```python
from build123d import *

# Parameters (mm, degrees)
BOSS_EXTRUDE1_DEPTH = 80
BOSS_EXTRUDE2_DEPTH = 350
BOSS_EXTRUDE3_DEPTH = 350
SKETCH4_R           = 11
CUT_EXTRUDE1_DEPTH  = 350


with BuildPart() as part:
    # Sketch1 → Boss-Extrude1 (new, symmetric)
    with BuildSketch(Plane.XY):
        Polygon((15, 15), (-15, 15), (-15, 35), (-45, 35), (-45, 25), (-25, 25), (-25, -25), (-45, -25), (-45, -35), (-15, -35), (-15, -15), (15, -15), (15, -35), (45, -35), (45, -25), (25, -25), (25, 25), (45, 25), (45, 35), (15, 35), align=None)
    extrude(amount=BOSS_EXTRUDE1_DEPTH, both=True)

    # Sketch2 → Boss-Extrude2 (add)
    with BuildSketch(Plane.XY.offset(80)):
        Polygon((-45, -25), (-45, -35), (-15, -35), (-15, 35), (-45, 35), (-45, 25), (-25, 25), (-25, -25), align=None)
        Polygon((15, 35), (45, 35), (45, 25), (25, 25), (25, -25), (45, -25), (45, -35), (15, -35), align=None)
    extrude(amount=BOSS_EXTRUDE2_DEPTH)

    # Sketch3 → Boss-Extrude3 (add)
    with BuildSketch(Plane(origin=(0, 0, -80), x_dir=(-1, 0, 0), z_dir=(0, 0, -1))):
        Polygon((-45, -25), (-45, -35), (-15, -35), (-15, 35), (-45, 35), (-45, 25), (-25, 25), (-25, -25), align=None)
        Polygon((45, 35), (15, 35), (15, -35), (45, -35), (45, -25), (25, -25), (25, 25), (45, 25), align=None)
    extrude(amount=BOSS_EXTRUDE3_DEPTH)

    # Sketch4 → Cut-Extrude1 (cut)
    with BuildSketch(Plane.ZY.offset(25)):
        with Locations(Location((-415, 0, 0), (0, 0, 270))):
            Circle(SKETCH4_R)
        with Locations(Location((415, 0, 0), (0, 0, 270))):
            Circle(SKETCH4_R)
    extrude(amount=-CUT_EXTRUDE1_DEPTH, mode=Mode.SUBTRACT)


solid = part.part
```
Can you work these out from the model? Positions are in its coordinate system, mm. A direction names the side the tool comes from. Coordinates: 2 decimals unless noted, no trailing zeros. Loops run counter-clockwise (first coordinate to the right, second up) from the corner with the lowest first, then second, coordinate; pieces in that order, holes last. Notation, with made-up numbers: (33.5, 23.5) -> (54.5, 23.5) arc R31 cw to (54.5, 60.5) -> close; hole circle Ø9 at (-21.75, 45.25). An arc over 180 degrees is marked (long way). Answer as a JSON object with one key per item and string values.
1) Thinking about a two-plate mould opening in Z: for faces 5 (the face through (-24, 0, 430)), 6 (the face through (19.93, 2.38, 404.26)), 7 (the face through (-35, -25, 6)), which applies, pulls with the +Z half, pulls with the -Z half, needs draft (parallel to the pull), parting line crosses it, or undercut?
Results:
{"face 5": "pulls with the +Z half", "face 6": "undercut", "face 7": "needs draft"}
2) For P1, Ø17.5, axis at y = 0, z = -415, coming from the +X side; P2, Ø21, axis at y = -8, z = 117.5, coming from the +X side; P3, Ø15, axis at x = 3.5, z = 30.5, coming from the +Y side; P4, Ø5, axis at x = 7, y = 14, coming from the -Z side, each with a flat end and sliding along its axis, tell me the tip position at first contact or that it passes through.
Results:
{"P1": "passes through", "P2": "stops at x = 25", "P3": "stops at y = 15", "P4": "stops at z = -80"}
3) Imagine slicing it at D-D (z = -415). Please give me the cut outline in (x, y).
Results:
{"outline": "(-45, -35) -> (-15, -35) -> (-15, -11) -> (-25, -11) -> (-25, -25) -> (-45, -25) -> close; (-45, 25) -> (-25, 25) -> (-25, 11) -> (-15, 11) -> (-15, 35) -> (-45, 35) -> close; (15, -35) -> (45, -35) -> (45, -25) -> (25, -25) -> (25, -11) -> (15, -11) -> close; (15, 11) -> (25, 11) -> (25, 25) -> (45, 25) -> (45, 35) -> (15, 35) -> close"}
4) Imagine slicing it at C-C (z = 351). Please give me the cut outline in (x, y).
Results:
{"outline": "(-45, -35) -> (-15, -35) -> (-15, 35) -> (-45, 35) -> (-45, 25) -> (-25, 25) -> (-25, -25) -> (-45, -25) -> close; (15, -35) -> (45, -35) -> (45, -25) -> (25, -25) -> (25, 25) -> (45, 25) -> (45, 35) -> (15, 35) -> close"}
5) Imagine slicing it at B-B (x = 33). Please give me the cut outline in (y, z).
Results:
{"outline": "(-35, -430) -> (-25, -430) -> (-25, 430) -> (-35, 430) -> close; (25, -430) -> (35, -430) -> (35, 430) -> (25, 430) -> close"}
6) Imagine slicing it at A-A (y = 0). Please give me the cut outline in (x, z), then the cut area to 3 significant figures.
Results:
{"outline": "(-25, -430) -> (-15, -430) -> (-15, -426) -> (-25, -426) -> close; (-25, -404) -> (-15, -404) -> (-15, -80) -> (15, -80) -> (15, -404) -> (25, -404) -> (25, 404) -> (15, 404) -> (15, 80) -> (-15, 80) -> (-15, 404) -> (-25, 404) -> close; (-25, 426) -> (-15, 426) -> (-15, 430) -> (-25, 430) -> close; (15, -430) -> (25, -430) -> (25, -426) -> (15, -426) -> close; (15, 426) -> (25, 426) -> (25, 430) -> (15, 430) -> close", "area": "21,100 mm^2"}
7) For faces 1 (the face through (0, -15, 1)), 2 (the face through (25, 0, 6)), 3 (the face through (0, 0, 80)), 4 (the face through (0, 15, 1)), which set-ups out of +Z, -Z, +X, -X, +Y, -Y let a thin tool reach every point of the face, with its end or its side?
Results:
{"face 1": "+Z, -Z, -Y", "face 2": "+Z, -Z, +X", "face 3": "+Z, +Y, -Y", "face 4": "+Z, -Z, +Y"}
8) If I drill on line 1 (Z direction, x = 19.25, y = 0); line 2 (X direction, y = -30, z = 263.5); line 3 (X direction, y = 24, z = 213.5), over which ranges is the centre line in solid material (lowest first)?
Results:
{"line 1": "z = -430 to -426, -404 to 404, 426 to 430", "line 2": "x = -45 to -15, 15 to 45", "line 3": "x = -25 to -15, 15 to 25"}
